Check sheet for the drawn part. Datum: minimum x, y, z corner. Units: mm. A direction names the side the tool comes from. Round coordinates to 2 decimals unless told otherwise and drop trailing zeros. Write each loop counter-clockwise with the first axis right and the second up, starting at its lowest first coordinate (ties: lowest second). Pieces come first, ordered by that corner, then holes. Notation, with made-up numbers: M 78.25,87.25 L 115.25,87.25 A18 ccw 115.25,110.25 Z; hole C 2.25,61.5 d1. An arc over 180 degrees is marked long. One line per item, written item: value. Start each with the question number.
Item 1: Thickness scan on probe 1 along Y at (x, z) = (5.95, 1.2); probe 2 along X at (y, z) = (7.25, 1.55); probe 3 along X at (y, z) = (3.25, 2.75). Record the ranges inside material, lowest first. Write a range as from..to.
Item 2: Tool access check on the marked faces 5, 6 and 7. Record the directions out of +Z, -Z, +X, -X, +Y, -Y that give a thin tool (end or side, any length) a straight path to the whole face; none if there is none.
Item 3: Gauge pin test, flat ends, axial feed: pin 1 (1 mm diameter, centred on y = 8.5, z = 1, fed in from +X); pin 2 (0.9 mm diameter, centred on y = 6, z = 1, fed in from -X). Record the tip position at first contact, or that the pin passes through.
Item 4: Section check A-A, the plane x = 5.95. Record the cut outline in (y, z).
Item 5: Section check B-B, the plane z = 2.1. Record the cut outline in (x, y).
Item 6: Section check C-C, the plane y = 2. Record the cut outline in (x, z) (1 decimal), then the cut area to 3 significant figures.
Item 7: Draft check along Y on the marked faces 1, 2, 3 and 4. Enter one of: +Y half, -Y half, draft (parallel to the pull), parting line (faces both ways), or undercut.
Item 8: Section check D-D, the plane x = 2.5. Record the cut outline in (y, z).
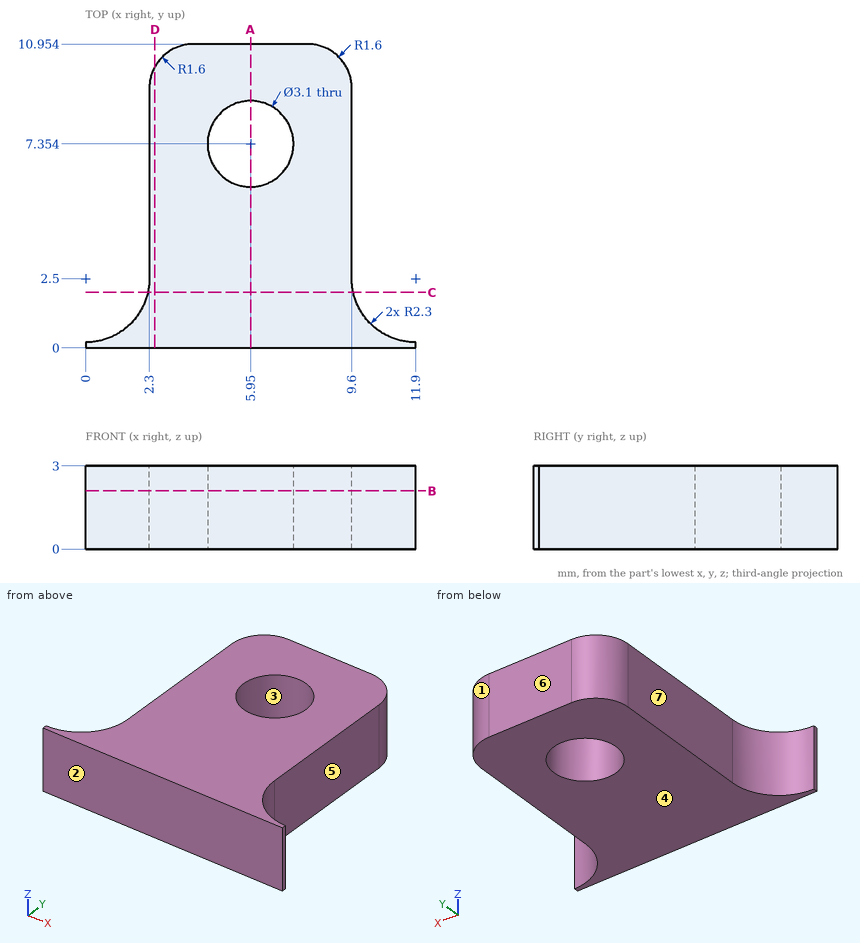
Response values:
1. probe 1: y = 0..5.8, 8.9..10.95
1. probe 2: x = 2.3..4.4, 7.5..9.6
1. probe 3: x = 2.3..9.6
2. face 5: +Z, -Z, +X, +Y
2. face 6: +Z, -Z, +X, -X, +Y
2. face 7: +Z, -Z, -X, +Y
3. pin 1: stops at x = 9.6
3. pin 2: stops at x = 2.3
4. outline: M 0,0 L 5.8,0 L 5.8,3 L 0,3 Z; M 8.9,0 L 10.95,0 L 10.95,3 L 8.9,3 Z
5. outline: M 0,0 L 11.9,0 L 11.9,0.2 A2.3 cw 9.6,2.5 L 9.6,9.35 A1.6 ccw 8,10.95 L 3.9,10.95 A1.6 ccw 2.3,9.35 L 2.3,2.5 A2.3 cw 0,0.2 Z; hole C 5.95,7.35 d3.1
6. outline: M 2.2,0 L 9.7,0 L 9.7,3 L 2.2,3 Z
6. area: 22.2 mm2
7. face 1: +Y half
7. face 2: -Y half
7. face 3: undercut
7. face 4: draft
8. outline: M 0,0 L 10.13,0 L 10.13,3 L 0,3 Z
